from build123d import *

# Parameters (mm, degrees)
CROQUIS1_R              = 6.35
CROQUIS1_W              = 92
CROQUIS1_H              = 92
SALIENTE_EXTRUIR1_DEPTH = 12.7


with BuildPart() as part:
    # Croquis1 → Saliente-Extruir1 (new body)
    with BuildSketch(Plane(origin=(0, 0, 0), x_dir=(1, 0, 0), z_dir=(0, 1, 0))):
        with BuildLine():
            Line((-109, 140), (109, 140))
            ThreePointArc((109, 140), (130.920310217, 130.920310217), (140, 109))
            Line((140, 109), (140, -109))
            ThreePointArc((140, -109), (130.920310217, -130.920310217), (109, -140))
            Line((109, -140), (-109, -140))
            ThreePointArc((-109, -140), (-130.920310217, -130.920310217), (-140, -109))
            Line((-140, -109), (-140, 109))
            ThreePointArc((-140, 109), (-130.920310217, 130.920310217), (-109, 140))
        make_face()
        with Locations((-109, -109)):
            Circle(CROQUIS1_R, mode=Mode.SUBTRACT)
        with Locations((-109, 109)):
            Circle(CROQUIS1_R, mode=Mode.SUBTRACT)
        with Locations((109, 109)):
            Circle(CROQUIS1_R, mode=Mode.SUBTRACT)
        with Locations((109, -109)):
            Circle(CROQUIS1_R, mode=Mode.SUBTRACT)
        Rectangle(CROQUIS1_W, CROQUIS1_H, mode=Mode.SUBTRACT)
    extrude(amount=SALIENTE_EXTRUIR1_DEPTH)


solid = part.part
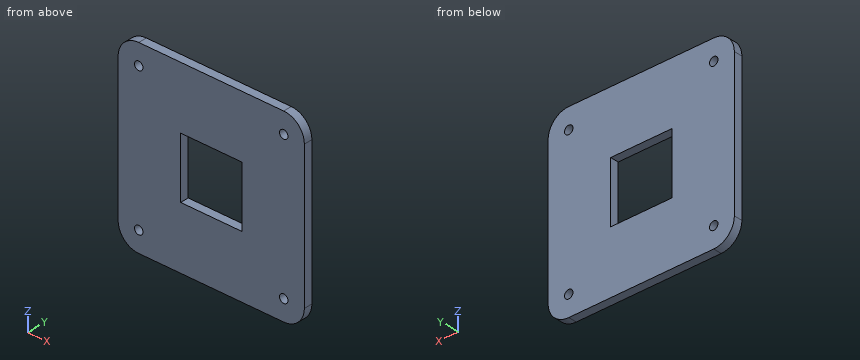
Geometry check sheet. Reference: the model listing, model coordinates, mm. Round coordinates to 2 decimals unless told otherwise and drop trailing zeros. Write each loop counter-clockwise with the first axis right and the second up, starting at its lowest first coordinate (ties: lowest second). Pieces come first, ordered by that corner, then holes.
Item 1: Section check A-A (x = 5). Record the boundary of the cut face in (y, z), plus the area to 3 significant figures.
Determined:
outline: (0, -140) - (12.7, -140) - (12.7, -46) - (0, -46) - close; (0, 46) - (12.7, 46) - (12.7, 140) - (0, 140) - close
area: 2,390 mm2
Item 2: Material ranges on line 1 along Z through (x, y) = (109, 7); line 2 along X through (y, z) = (2.25, -24), recorded low to high.
Determined:
line 1: z = -140 to -115.35, -102.65 to 102.65, 115.35 to 140
line 2: x = -140 to -46, 46 to 140
Item 3: Section check B-B (z = 25). Record the boundary of the cut face in (x, y).
Determined:
outline: (-140, 0) - (-46, 0) - (-46, 12.7) - (-140, 12.7) - close; (46, 0) - (140, 0) - (140, 12.7) - (46, 12.7) - close
Item 4: Section check C-C (y = 4). Record the boundary of the cut face in (x, z), plus the area to 3 significant figures.
Determined:
outline: (-140, -109) arc R31 ccw to (-109, -140) - (109, -140) arc R31 ccw to (140, -109) - (140, 109) arc R31 ccw to (109, 140) - (-109, 140) arc R31 ccw to (-140, 109) - close; hole circle Ø12.7 at (-109, -109); hole circle Ø12.7 at (-109, 109); hole (-46, -46) - (46, -46) - (46, 46) - (-46, 46) - close; hole circle Ø12.7 at (109, -109); hole circle Ø12.7 at (109, 109)
area: 68,600 mm2
